CAD build for the part. Positions are in the model's coordinates, mm. A direction names the side the tool comes from. Give positions to 0.01 mm unless a question says otherwise; leave off trailing zeros. Order: outer loops, then holes, each group sorted by start corner. A loop starts at its lowest first (then second) coordinate and runs counter-clockwise, first axis right, second up.
from build123d import *

# Parameters (mm, degrees)
F1_DEPTH = 63.5
F2_DEPTH = 25.4
F3_DEPTH = 12.7


with BuildPart() as f1:
    # F0 (on Front) → F1 (new body, symmetric)
    with BuildSketch(Plane.XZ):
        Polygon((-41.275, -9.525), (41.275, -9.525), (41.275, 9.525), (22.225, 9.525), (-41.275, 9.525), align=None)
    extrude(amount=F1_DEPTH, both=True)

    # F0 (on Front) → F2 (join, symmetric)
    with BuildSketch(Plane.XZ):
        with BuildLine():
            Line((22.225, 9.525), (41.275, 9.525))
            Line((41.275, 9.525), (41.275, 27.0002))
            ThreePointArc((41.275, 27.0002), (45.9246798487, 38.2255201513), (57.15, 42.8752))
            Line((57.15, 42.8752), (60.4529731631, 42.8752))
            Line((60.4529731631, 42.8752), (60.4529731631, 61.938414402))
            Line((60.4529731631, 61.938414402), (57.15, 61.9252))
            ThreePointArc((57.15, 61.9252), (32.4542956671, 51.6959043329), (22.225, 27.0002))
            Line((22.225, 27.0002), (22.225, 9.525))
        make_face()
        Polygon((85.7571963739, 62.0396505186), (60.4529731631, 61.938414402), (60.4529731631, 42.8752), (85.8338687354, 42.8752), align=None)
    extrude(amount=F2_DEPTH, both=True)

    # F0 (on Front) → F3 (join, symmetric)
    with BuildSketch(Plane.XZ):
        with BuildLine():
            add(Edge.make_bspline(
                [(-41.275, 9.525), (-41.2464402616, 42.1838574111), (8.0350227654, 62.539242208), (57.15, 61.9252)],
                knots=[0, 0, 0, 0, 111.5045361635, 111.5045361635, 111.5045361635, 111.5045361635], degree=3))
            Line((-41.275, 9.525), (22.225, 9.525))
            Line((22.225, 9.525), (22.225, 27.0002))
            ThreePointArc((22.225, 27.0002), (32.4542956671, 51.6959043329), (57.15, 61.9252))
        make_face()
    extrude(amount=F3_DEPTH, both=True)

    # F0 (on Front) → F4 (revolve)
    with BuildSketch(Plane.XZ):
        Polygon((85.7386514544, 66.675), (85.7571963739, 62.0396505186), (85.8338687354, 42.8752), (85.8529731631, 38.1), (111.2529731631, 38.1), (111.2529731631, 66.675), align=None)
    revolve(axis=Axis((85.7958123088, 0, 52.3875), (0.0040007277, 0, -0.9999919971)))


solid = f1.part
1. Wall check: line 1 (Z direction, x = 27.5, y = 54.5) (3 decimals); line 2 (X direction, y = -5, z = -1) (3 decimals); line 3 (Z direction, x = 21, y = 11) (3 decimals). Give the ranges that are in metal, low to high.
2. Saw through at A-A on z = -1.5. Give the cut face in (x, y) (3 decimals).
3. Mould opens along X. For faces 1 (the flat face through (-2, 12.7, 31)), 2 (the flat face through (41.275, -1, 4)), 3 (the conical face through (110.077, -7.647, 52.583)) say: released by +X, released by -X, zero draft, split by the parting line, or undercut.
4. 3-axis set-ups, long thin cutter, end or side, ignore diameter. For faces 4 (the cylindrical face through (45.8, -0.4, 38.1)), 5 (the cylindrical face through (32.73, 18.96, 51.97)): which of +Z, -Z, +X, -X, +Y, -Y reach the whole face in a straight line?
5. Pin check, flat tips, straight feed: P1, Ø10, axis at x = 77.5, z = 35, coming from the -Y side; P2, Ø1, axis at y = -9.5, z = 20, coming from the -X side; P3, Ø8, axis at x = 58.5, z = 54.5, coming from the +Y side. Stop position of each tip, or through.
6. Saw through at B-B on y = -47. Give the cut face in (x, z) (3 decimals).
Reported:
1. line 1: z = -9.525 to 9.525
1. line 2: x = -41.275 to 41.275
1. line 3: z = -9.525 to 58.578
2. outline: (-41.275, -63.5) - (41.275, -63.5) - (41.275, 63.5) - (-41.275, 63.5) - close
3. face 1: zero draft
3. face 2: released by +X
3. face 3: undercut
4. face 4: -Z, +Y, -Y
4. face 5: +Z, -X, +Y
5. P1: stops at y = -25.03
5. P2: stops at x = -39.66
5. P3: stops at y = 25.4
6. outline: (-41.275, -9.525) - (41.275, -9.525) - (41.275, 9.525) - (-41.275, 9.525) - close
